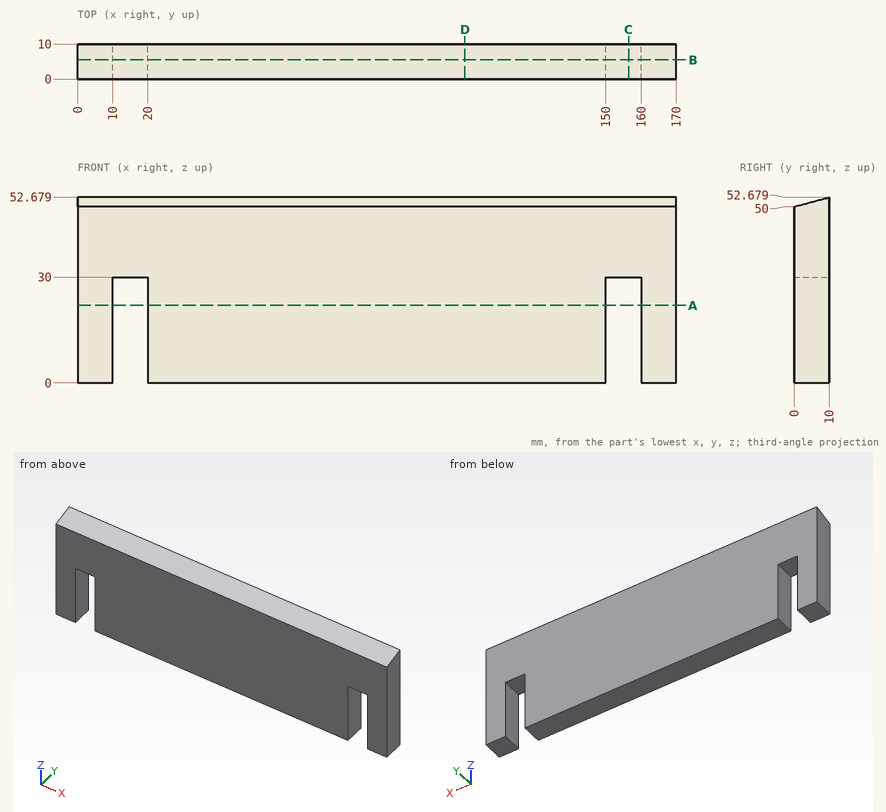
Here's the drawing with two shaded views (mm, measured from the low corner). I have some questions. Give positions to 0.01 mm unless a question says otherwise; leave off trailing zeros. Loops run counter-clockwise (first coordinate to the right, second up) from the corner with the lowest first, then second, coordinate; pieces in that order, holes last. Notation, with made-up numbers: M 37.5,71.5 L 62.5,71.5 A14 ccw 62.5,82.5 Z; hole C 36.25,-18.5 d3. An arc over 180 degrees is marked long. Answer in a Markdown table with one row per item.
1. Suppose I cut it at B-B on y = 5.5. Write out the boundary of the cut face in (x, z), plus the area to 3 significant figures.
Taken from the geometry:
| item | result |
|---|---|
| outline | M 0,0 L 10,0 L 10,30 L 20,30 L 20,0 L 150,0 L 150,30 L 160,30 L 160,0 L 170,0 L 170,51.47 L 0,51.47 Z |
| area | 8,150 mm² |
2. Suppose I cut it at A-A on z = 22. Write out the boundary of the cut face in (x, y).
Taken from the geometry:
| item | result |
|---|---|
| outline | M 0,0 L 10,0 L 10,10 L 0,10 Z; M 20,0 L 150,0 L 150,10 L 20,10 Z; M 160,0 L 170,0 L 170,10 L 160,10 Z |
3. Suppose I cut it at D-D on x = 110. Write out the boundary of the cut face in (y, z).
Taken from the geometry:
| item | result |
|---|---|
| outline | M 0,0 L 10,0 L 10,52.68 L 0,50 Z |
4. If I drill on line 1 along X through (y, z) = (4, 28.5); line 2 along Z through (x, y) = (93, 8.5); line 3 along Z through (x, y) = (130.5, 6), over which ranges is the centre line in solid material (lowest first)?
Taken from the geometry:
| item | result |
|---|---|
| line 1 | x = 0 to 10, 20 to 150, 160 to 170 |
| line 2 | z = 0 to 52.28 |
| line 3 | z = 0 to 51.61 |
5. Suppose I cut it at C-C on x = 156.5. Write out the boundary of the cut face in (y, z), plus the area to 3 significant figures.
Taken from the geometry:
| item | result |
|---|---|
| outline | M 0,30 L 10,30 L 10,52.68 L 0,50 Z |
| area | 213 mm² |
6. For pin 1 Ø1 at (y, z) = (8, 17) entering from -X; pin 2 Ø3 at (x, y) = (17, 4) entering from -Z, each with a flat end and sliding along its axis, tell me the tip position at first contact or that it passes through.
Taken from the geometry:
| item | result |
|---|---|
| pin 1 | stops at x = 0 |
| pin 2 | stops at z = 30 |
